```python
from build123d import *

# Parameters (mm, degrees)
SKETCH_1_W                   = 7
SKETCH_1_H                   = 40
EXTRUDE_1_DEPTH              = 4.8
HOLE_WIZARD_M2_1_D           = 2.4
HOLE_WIZARD_M2_1_DEPTH       = 10.1
HOLE_WIZARD_M2_1_CBORE_D     = 4.4
HOLE_WIZARD_M2_1_CBORE_DEPTH = 2.4
HOLE_WIZARD_M2_1_TIP         = 0.721032743


with BuildPart() as part:
    # 草图1 → 凸台-拉伸1 (new body)
    with BuildSketch(Plane.XY):
        with Locations((3.5, 20)):
            Rectangle(SKETCH_1_W, SKETCH_1_H)
    extrude(amount=EXTRUDE_1_DEPTH)

    # M2 六角凹头螺钉的柱形沉头孔1
    with Locations(Plane.XY.offset(4.8)):
        with Locations((3.5, 35), (3.5, 20), (3.5, 5)):
            CounterBoreHole(HOLE_WIZARD_M2_1_D / 2, HOLE_WIZARD_M2_1_CBORE_D / 2, HOLE_WIZARD_M2_1_CBORE_DEPTH, depth=HOLE_WIZARD_M2_1_DEPTH)
            with Locations((0, 0, -(HOLE_WIZARD_M2_1_DEPTH + HOLE_WIZARD_M2_1_TIP / 2))):  # 118° drill point
                Cone(0, HOLE_WIZARD_M2_1_D / 2, HOLE_WIZARD_M2_1_TIP, mode=Mode.SUBTRACT)


solid = part.part
```
Verification items for the finished model (mm, model axes). A direction names the side the tool comes from. Round coordinates to 2 decimals unless told otherwise and drop trailing zeros. Order: outer loops, then holes, each group sorted by start corner. A loop starts at its lowest first (then second) coordinate and runs counter-clockwise, first axis right, second up. Notation, with made-up numbers: (66.25, 71) - (72.25, 71) arc R14 cw to (72.25, 75) - close; hole circle Ø10 at (-33.75, -27.5). An arc over 180 degrees is marked (long way). Use CSV: the item, a comma, the result in double quotes. Start each with the question number.
1) Section check A-A, the plane x = 3.5. Record the cut outline in (y, z).
2) Go/stop test with flat-tipped pins: P1, Ø3.5, axis at x = 3.5, y = 35, coming from the +Z side; P2, Ø3, axis at x = 3.5, y = 5, coming from the -Z side. Record where each tip stops, or that it passes through.
3) Section check B-B, the plane y = 5. Record the cut outline in (x, z).
4) Mould release check, pull along X, two halves, no side actions. Record for faces 3 (the flat face through (5, 35, 2.4)), 4 (the flat face through (1, 20, 4.8)), 5 (the flat face through (0, 20, 2)): +X half, -X half, draft (parallel to the pull), parting line (faces both ways), or undercut.
5) Thickness scan on L1, parallel to Y at x = 3.5, z = 1.5; L2, parallel to Y at x = 3.5, z = 3.8; L3, parallel to X at y = 35.5, z = 4.2. Record the ranges inside material, lowest first.
6) Access from +Z, -Z, +X, -X, +Y, -Y to the whole of each face (thin tool, end or side, straight path). Record for faces 1 (the cylindrical face through (3.023, 32.852, 3.617)), 2 (the flat face through (5, 20, 0)).
7) Section check D-D, the plane y = 19.5. Record the cut outline in (x, z).
8) Section check C-C, the plane z = 3.7. Record the cut outline in (x, y), plus the area to 3 significant figures.
Answers:
1,outline,"(0, 0) - (3.8, 0) - (3.8, 2.4) - (2.8, 2.4) - (2.8, 4.8) - (0, 4.8) - close; (6.2, 0) - (18.8, 0) - (18.8, 2.4) - (17.8, 2.4) - (17.8, 4.8) - (7.2, 4.8) - (7.2, 2.4) - (6.2, 2.4) - close; (21.2, 0) - (33.8, 0) - (33.8, 2.4) - (32.8, 2.4) - (32.8, 4.8) - (22.2, 4.8) - (22.2, 2.4) - (21.2, 2.4) - close; (36.2, 0) - (40, 0) - (40, 4.8) - (37.2, 4.8) - (37.2, 2.4) - (36.2, 2.4) - close"
2,P1,"stops at z = 2.4"
2,P2,"stops at z = 0"
3,outline,"(0, 0) - (2.3, 0) - (2.3, 2.4) - (1.3, 2.4) - (1.3, 4.8) - (0, 4.8) - close; (4.7, 0) - (7, 0) - (7, 4.8) - (5.7, 4.8) - (5.7, 2.4) - (4.7, 2.4) - close"
4,face 3,"undercut"
4,face 4,"draft"
4,face 5,"-X half"
5,L1,"y = 0 to 3.8, 6.2 to 18.8, 21.2 to 33.8, 36.2 to 40"
5,L2,"y = 0 to 2.8, 7.2 to 17.8, 22.2 to 32.8, 37.2 to 40"
5,L3,"x = 0 to 1.36, 5.64 to 7"
6,face 1,"+Z"
6,face 2,"-Z, +X, -X, +Y, -Y"
7,outline,"(0, 0) - (2.41, 0) - (2.41, 2.4) - (1.36, 2.4) - (1.36, 4.8) - (0, 4.8) - close; (4.59, 0) - (7, 0) - (7, 4.8) - (5.64, 4.8) - (5.64, 2.4) - (4.59, 2.4) - close"
8,outline,"(0, 0) - (7, 0) - (7, 40) - (0, 40) - close; hole circle Ø4.4 at (3.5, 5); hole circle Ø4.4 at (3.5, 20); hole circle Ø4.4 at (3.5, 35)"
8,area,"234 mm²"
